```python
from build123d import *

# Parameters (mm, degrees)
SKETCH_1_W          = 36
SKETCH_1_H          = 42
EXTRUDE_1_DEPTH     = 2
SKETCH_2_R          = 1.75
SKETCH_2_R_2        = 2.5
CUT_EXTRUDE_1_DEPTH = 56.353410012
SKETCH_3_R          = 4
CUT_EXTRUDE_2_DEPTH = 56.353410012


with BuildPart() as part:
    # 草图1 → 凸台-拉伸1 (new body)
    with BuildSketch(Plane.XY):
        with Locations((18, 21)):
            Rectangle(SKETCH_1_W, SKETCH_1_H)
    extrude(amount=EXTRUDE_1_DEPTH)

    # 草图2 → 切除-拉伸1 (cut, through all)
    with BuildSketch(Plane.XY.offset(2)):
        with Locations((32.5, 38.5)):
            Circle(SKETCH_2_R)
        with Locations((22.5, 28)):
            Circle(SKETCH_2_R)
        with Locations((10.5, 35.5)):
            Circle(SKETCH_2_R_2)
    extrude(amount=-CUT_EXTRUDE_1_DEPTH, mode=Mode.SUBTRACT)

    # 草图3 → 切除-拉伸2 (cut, through all)
    with BuildSketch(Plane.XY.offset(2)):
        with Locations((10.5, 8.5)):
            Circle(SKETCH_3_R)
    extrude(amount=-CUT_EXTRUDE_2_DEPTH, mode=Mode.SUBTRACT)


solid = part.part
```
Work out the finished part from the listing and answer in its coordinate system (mm). Give positions to 0.01 mm unless a question says otherwise; leave off trailing zeros. Loops run counter-clockwise (first coordinate to the right, second up) from the corner with the lowest first, then second, coordinate; pieces in that order, holes last. Notation, with made-up numbers: (12.5, 74.5) - (32.5, 74.5) arc R6 ccw to (32.5, 80.5) - close; hole circle Ø5 at (19, -23). An arc over 180 degrees is marked (long way). One line per question, with ' | ' between items.
(1) The part is cut by section B-B (x = 22.5). Write down the section's boundary in (y, z).
Recorded:
outline: (0, 0) - (26.25, 0) - (26.25, 2) - (0, 2) - close; (29.75, 0) - (42, 0) - (42, 2) - (29.75, 2) - close
(2) The part is cut by section A-A (y = 35.5). Write down the section's boundary in (x, z), then the cut area to 3 significant figures.
Recorded:
outline: (0, 0) - (8, 0) - (8, 2) - (0, 2) - close; (13, 0) - (36, 0) - (36, 2) - (13, 2) - close | area: 62.0 mm²
(3) Straight lines are drawn through the part: probe 1 along Y at (x, z) = (10.5, 1.5); probe 2 along Y at (x, z) = (32.5, 1.5); probe 3 along Y at (x, z) = (9.5, 0.25). For each, find the intervals that lie inside material, in ascending order.
Recorded:
probe 1: y = 0 to 4.5, 12.5 to 33, 38 to 42 | probe 2: y = 0 to 36.75, 40.25 to 42 | probe 3: y = 0 to 4.63, 12.37 to 33.21, 37.79 to 42
(4) The part is cut by section D-D (z = 1.45). Write down the section's boundary in (x, y), then the cut area to 3 significant figures.
Recorded:
outline: (0, 0) - (36, 0) - (36, 42) - (0, 42) - close; hole circle Ø8 at (10.5, 8.5); hole circle Ø5 at (10.5, 35.5); hole circle Ø3.5 at (22.5, 28); hole circle Ø3.5 at (32.5, 38.5) | area: 1,420 mm²
(5) The part is cut by section C-C (x = 10.5). Write down the section's boundary in (y, z), then the cut area to 3 significant figures.
Recorded:
outline: (0, 0) - (4.5, 0) - (4.5, 2) - (0, 2) - close; (12.5, 0) - (33, 0) - (33, 2) - (12.5, 2) - close; (38, 0) - (42, 0) - (42, 2) - (38, 2) - close | area: 58.0 mm²
(6) The mould has two halves that part along Y. Classify faces 1 (the face through (9.96, 33.06, 1.01)), 2 (the face through (18, 21, 2)), 3 (the face through (18, 0, 1)): +Y half, -Y half, draft (parallel to the pull), parting line (faces both ways), or undercut.
Recorded:
face 1: undercut | face 2: draft | face 3: -Y half
